```python
from build123d import *

# Parameters (mm, degrees)
CHAMFER_1_SIZE      = 0.5
CUT_EXTRUDE_1_DEPTH = 1.2
SKETCH_5_R          = 4
CUT_EXTRUDE_2_DEPTH = 5
CUT_EXTRUDE_3_DEPTH = 1.2


with BuildPart() as part:
    # Sketch 1 → Revolve 1 (revolve)
    with BuildSketch(Plane.XY, mode=Mode.PRIVATE) as revolve_1_sk:
        with BuildLine():
            Line((0, 2.5), (0, 0))
            Line((0, 0), (721.167070453, 0))
            Line((721.167070453, 0), (1185.852894625, 0))
            Line((1185.852894625, 0), (2359.852894625, 0))
            Line((2359.852894625, 0), (2410.852894625, 0))
            Line((2410.852894625, 0), (2410.852894625, 3))
            Line((2410.852894625, 3), (2375.852894625, 3))
            Line((2375.852894625, 3), (2375.852894625, 10))
            Line((2375.852894625, 10), (2359.852894625, 10))
            Line((2359.852894625, 10), (1206.852894625, 10))
            Line((1206.852894625, 10), (1185.852894625, 10))
            Line((1185.852894625, 10), (1145.2, 10))
            ThreePointArc((1145.2, 10), (1145.058578644, 10.058578644), (1145, 10.2))
            Line((1145, 10.2), (1145, 10.5))
            Line((1145, 10.5), (1144.5, 11))
            Line((1144.5, 11), (51.5, 11))
            Line((51.5, 11), (51, 10.5))
            Line((51, 10.5), (51, 10.2))
            ThreePointArc((51, 10.2), (50.941421356, 10.058578644), (50.8, 10))
            Line((50.8, 10), (35.5, 10))
            Line((35.5, 10), (35, 9.5))
            Line((35, 9.5), (35, 3.5))
            ThreePointArc((35, 3.5), (34.853553391, 3.146446609), (34.5, 3))
            Line((34.5, 3), (0.5, 3))
            Line((0.5, 3), (0, 2.5))
        make_face()
    revolve(revolve_1_sk.sketch.rotate(Axis((0, 0, 0), (1, 0, 0)), 90), axis=Axis((0, 0, 0), (1, 0, 0)))

    # Chamfer 1
    chamfer_1_edges = [part.edges().sort_by_distance(p)[0] for p in [
        (2375.852894625, 0, -10),
        (2410.852894625, 0, -3),
    ]]
    chamfer(chamfer_1_edges, length=CHAMFER_1_SIZE)

    # Sketch 3 → Cut-Extrude 1 (cut)
    with BuildSketch(Plane.XY.offset(10)):
        with BuildLine():
            Line((39, 3), (47, 3))
            ThreePointArc((47, 3), (50, 0), (47, -3))
            Line((47, -3), (39, -3))
            ThreePointArc((39, -3), (36, 0), (39, 3))
        make_face()
    extrude(amount=-CUT_EXTRUDE_1_DEPTH, mode=Mode.SUBTRACT)

    # Sketch 5 → Cut-Extrude 2 (cut)
    with BuildSketch(Plane(origin=(0, 0, -10), x_dir=(-1, 0, 0), z_dir=(0, 0, -1))):
        with Locations((-1155, 0)):
            Circle(SKETCH_5_R)
    extrude(amount=-CUT_EXTRUDE_2_DEPTH, mode=Mode.SUBTRACT)

    # Sketch 6 → Cut-Extrude 3 (cut)
    with BuildSketch(Plane.XY.offset(10)):
        with BuildLine():
            Line((2363.852894625, 3), (2371.852894625, 3))
            ThreePointArc((2371.852894625, 3), (2374.852894625, 0), (2371.852894625, -3))
            Line((2371.852894625, -3), (2363.852894625, -3))
            ThreePointArc((2363.852894625, -3), (2360.852894625, 0), (2363.852894625, 3))
        make_face()
    extrude(amount=-CUT_EXTRUDE_3_DEPTH, mode=Mode.SUBTRACT)


solid = part.part
```
The model under review builds one solid part; all positions refer to its coordinate system, in mm. Round coordinates to 2 decimals unless told otherwise and drop trailing zeros. Write each loop counter-clockwise with the first axis right and the second up, starting at its lowest first coordinate (ties: lowest second). Pieces come first, ordered by that corner, then holes. Notation, with made-up numbers: M 31,82.25 L 79,82.25 A31 ccw 79,121.25 Z; hole C 85,23 d3. An arc over 180 degrees is marked long. Use CSV: the item, a comma, the result in double quotes. Start each with the question number.
(1) Clearance check with flat-ended pins moving along their axes: P1, Ø10, axis at x = 975.5, z = -8.5, coming from the +Y side; P2, Ø1.8, axis at x = 2366.5, y = -1, coming from the +Z side; P3, Ø2, axis at y = 5, z = -8, coming from the +X side; P4, Ø5.5, axis at y = -1.5, z = 3, coming from the +X side. State where each tip first meets the part, or that it passes through.
(2) We need section B-B, the plane x = 954. State the section outline as (y, z) points, then the cut area to 3 significant figures.
(3) For line 1 along X through (y, z) = (0, -7); line 2 along Y through (x, z) = (808, -0.75); line 3 along Y through (x, z) = (738.5, -3.75), list the stretches that pass through material, from the lowest coordinate up.
(4) We need section A-A, the plane x = 1776. State the section outline as (y, z) points.
Findings:
1,P1,"y = 10.43"
1,P2,"z = 8.8"
1,P3,"x = 2375.85"
1,P4,"x = 2410.85"
2,outline,"C 0,0 d22"
2,area,"380 mm^2"
3,line 1,"35 to 1151, 1159 to 2375.85"
3,line 2,"-10.97 to 10.97"
3,line 3,"-10.34 to 10.34"
4,outline,"C 0,0 d20"
